from build123d import *

# Parameters (mm, degrees)
SKETCH_R     = 7.75
SKETCH_R_2   = 6.3
PAD_DEPTH    = 1.125
CHAMFER_SIZE = 0.25


with BuildPart() as part:
    # Sketch → Pad (new body)
    with BuildSketch(Plane.XY):
        Circle(SKETCH_R)
        Circle(SKETCH_R_2, mode=Mode.SUBTRACT)
    extrude(amount=PAD_DEPTH)

    # Chamfer
    chamfer_edges = [part.edges().sort_by_distance(p)[0] for p in [
        (-7.75, 0, 1.125),
        (-6.3, 0, 1.125),
        (-7.75, 0, 0),
        (-6.3, 0, 0),
    ]]
    chamfer(chamfer_edges, length=CHAMFER_SIZE)


solid = part.part
Can you work these out from the model? Positions are in its coordinate system, mm. Give positions to 0.01 mm unless a question says otherwise; leave off trailing zeros. Loops run counter-clockwise (first coordinate to the right, second up) from the corner with the lowest first, then second, coordinate; pieces in that order, holes last. Notation, with made-up numbers: M -35,26 L 0,26 A20 ccw 0,58 Z; hole C 85.5,32.5 d2. An arc over 180 degrees is marked long. One line per item, written item: value. Start each with the question number.
1) I'm going to push a flat-ended pin straight in: pin 1 (5 mm diameter, centred on x = 1.5, y = 5, fed in from -Z). Where does the tip first touch, or does it pass through?
2) Thinking about a two-plate mould opening in X: for faces 1 (the face through (-5, -3.83, 0.56)), 2 (the face through (-1.009, 7.684, 0.558)), 3 (the face through (0, -7, 1.125)), which applies, +X half, -X half, draft (parallel to the pull), parting line (faces both ways), or undercut?
3) If we section it at C-C, the plane z = 0.6: Write out the boundary of the cut face in (x, y).
4) If I drill on line 1 (Y direction, x = -0.25, z = 0.75); line 2 (Y direction, x = 3.75, z = 0.2); line 3 (X direction, y = 5, z = 0.35), over which ranges is the centre line in solid material (lowest first)? Write a range as [from, to].
5) If we section it at A-A, the plane x = 0: Write out the boundary of the cut face in (y, z) (3 decimals).
Completed:
1. pin 1: stops at z = 0
2. face 1: undercut
2. face 2: parting line
2. face 3: draft
3. outline: C 0,0 d15.5; hole C 0,0 d12.6
4. line 1: y = [-7.75, -6.3], [6.3, 7.75]
4. line 2: y = [-6.73, -5.12], [5.12, 6.73]
4. line 3: x = [-5.92, -3.83], [3.83, 5.92]
5. outline: M -7.75,0.25 L -7.5,0 L -6.55,0 L -6.3,0.25 L -6.3,0.875 L -6.55,1.125 L -7.5,1.125 L -7.75,0.875 Z; M 6.3,0.25 L 6.55,0 L 7.5,0 L 7.75,0.25 L 7.75,0.875 L 7.5,1.125 L 6.55,1.125 L 6.3,0.875 Z
